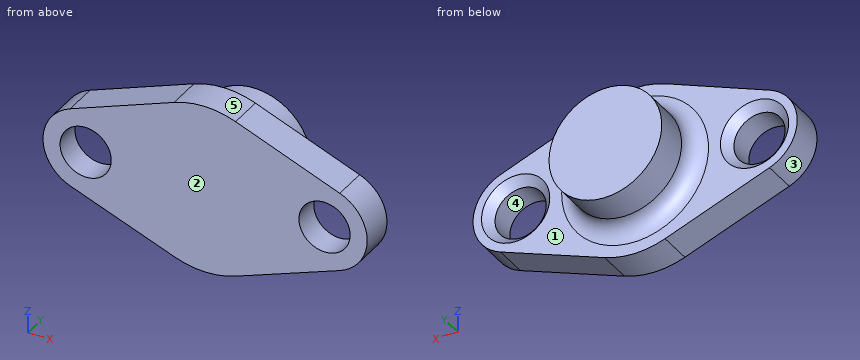
from build123d import *

# Parameters (mm, degrees)
EXTRUDE_316_DEPTH   = 20
SKETCH_2_R          = 33.033320501
EXTRUDE_1_DEPTH     = 30
SKETCH_3_R          = 15
CUT_EXTRUDE_1_DEPTH = 112.46747736
FILLET_1_R          = 10
CHAMFER_1_SIZE      = 5


with BuildPart() as part:
    # Эскиз1 → Extrude 316 (new body)
    with BuildSketch(Plane(origin=(0, 0, 0), x_dir=(-1, 0, 0), z_dir=(0, -1, 0))):
        with BuildLine():
            Line((-78.917505692, 23.388614652), (-17.835027079, 46.710938859))
            ThreePointArc((-17.835027079, 46.710938859), (-0.148812417, 49.999778548), (17.556665634, 46.816273793))
            Line((17.556665634, 46.816273793), (78.776887546, 23.857954408))
            ThreePointArc((78.776887546, 23.857954408), (94.998038561, 0.610466623), (79.076996078, -22.84357002))
            Line((79.076996078, -22.84357002), (18.156882698, -46.586775062))
            ThreePointArc((18.156882698, -46.586775062), (0.148812417, -49.999778548), (-17.879254632, -46.694028031))
            Line((-17.879254632, -46.694028031), (-78.939619469, -23.313868793))
            ThreePointArc((-78.939619469, -23.313868793), (-94.99998935, 0.044982802), (-78.917505692, 23.388614652))
        make_face()
    extrude(amount=EXTRUDE_316_DEPTH)

    # Эскиз2 → Бобышка-Вытянуть1 (add)
    with BuildSketch(Plane(origin=(0, 0, 0), x_dir=(-1, 0, 0), z_dir=(0, 1, 0))):
        with Locations(Location((0, 0, 0), (0, 0, 180))):
            Circle(SKETCH_2_R)
    extrude(amount=EXTRUDE_1_DEPTH)

    # Эскиз3 → Вырез-Вытянуть1 (cut, through all)
    with BuildSketch(Plane(origin=(0, 0, 0), x_dir=(-1, 0, 0), z_dir=(0, 1, 0))):
        with Locations((-69.999992153, -0.033145222)):
            Circle(SKETCH_3_R)
        with Locations((69.998554729, -0.449817511)):
            Circle(SKETCH_3_R)
    extrude(amount=-CUT_EXTRUDE_1_DEPTH, mode=Mode.SUBTRACT)

    # Скругление1
    fillet_1_edges = [part.edges().sort_by_distance(p)[0] for p in [
        (-33.033320501, 0, 0),
    ]]
    fillet(fillet_1_edges, radius=FILLET_1_R)

    # Фаска1
    chamfer_1_edges = [part.edges().sort_by_distance(p)[0] for p in [
        (84.999992153, 0, -0.033145222),
        (-54.998554729, 0, -0.449817511),
    ]]
    chamfer(chamfer_1_edges, length=CHAMFER_1_SIZE)


solid = part.part
Source: CAD feature listing. Evaluate the final solid. Frame: model axes, mm. Face numbers are marked on the shaded views. A direction names the side the tool comes from. Coordinates: 2 decimals unless noted, no trailing zeros. Loops run counter-clockwise (first coordinate to the right, second up) from the corner with the lowest first, then second, coordinate; pieces in that order, holes last. Notation, with made-up numbers: M 20.5,5 L 53.5,5 A22 cw 53.5,34 Z; hole C 41.5,-2 d10. An arc over 180 degrees is marked long. Answer in a Markdown table with one row per item.
Q1. Ray query, probe 1 along Y at (x, z) = (46, -7.5); probe 2 along Z at (x, y) = (69, -2); probe 3 along X at (y, z) = (24.5, -26). Return the intervals inside material, ascending. Write a range as from..to.
Answers below:
| item | result |
|---|---|
| probe 1 | y = -20..0 |
| probe 2 | z = -27.18..-18.01, 17.94..27.12 |
| probe 3 | x = -20.38..20.38 |
Q2. Section B-B on y = 22.5. Return the cut outline in (x, z), plus the area to 3 significant figures.
Answers below:
| item | result |
|---|---|
| outline | C 0,0 d66.07 |
| area | 3,430 mm^2 |
Q3. Section C-C on z = -8.5. State how many separate pieces and enclosed holes the cut face has, plus the area to 3 significant figures.
Answers below:
| item | result |
|---|---|
| separate pieces | 3 |
| enclosed holes | 0 |
| area | 4,640 mm^2 |
Q4. Draft query along X for the marked faces 3, 4 and 5. Return one class per face: pulls with the +X half, pulls with the -X half, needs draft (parallel to the pull), parting line crosses it, or undercut.
Answers below:
| item | result |
|---|---|
| face 3 | pulls with the -X half |
| face 4 | undercut |
| face 5 | parting line crosses it |
Q5. First-contact query: pin 1 (2 mm diameter, centred on y = 12.5, z = -25, fed in from +X); pin 2 (5 mm diameter, centred on y = 18.5, z = -18.5, fed in from +X); pin 3 (10 mm diameter, centred on y = -3.5, z = -27, fed in from -X). Flat tips, straight axial feed; report the tip coordinate or a pass-through.
Answers below:
| item | result |
|---|---|
| pin 1 | stops at x = 22.7 |
| pin 2 | stops at x = 28.9 |
| pin 3 | stops at x = -82.67 |
Q6. Set-up query: the marked faces 1 and 2. Return all of +Z, -Z, +X, -X, +Y, -Y with unobstructed straight access to the full face (end or side cutting, diameter ignored); none if empty.
Answers below:
| item | result |
|---|---|
| face 1 | +Y |
| face 2 | +Z, -Z, +X, -X, -Y |
Q7. Section A-A on x = 0. Return the cut outline in (y, z).
Answers below:
| item | result |
|---|---|
| outline | M -20,-50 L 0,-50 L 0,-43.03 A10 cw 10,-33.03 L 30,-33.03 L 30,33.03 L 10,33.03 A10 cw 0,43.03 L 0,50 L -20,50 Z |
